Solid Edge part; units mm, degrees
sketch "Sketch1" plane through (0, 0, 0) normal (0, 0, 1) x (1, 0, 0)
  line L0 (70, -35) -> (70, 35)
  line L1 (70, 35) -> (34, 35)
  line L2 (34, 35) -> (34, 105)
  line L3 (34, 105) -> (-34, 105)
  line L4 (-34, 105) -> (-34, 35)
  line L5 (-34, 35) -> (-70, 35)
  line L6 (-70, 35) -> (-70, -35)
  line L7 (-40, -35) -> (-70, -35)
  line L8 (-40, -80) -> (-40, -35)
  line L9 (40, -80) -> (-40, -80)
  line L10 (40, -35) -> (40, -80)
  line L11 (70, -35) -> (40, -35)
  dimension "D1" = 70
  dimension "D2" = 70
  dimension "D3" = 40
  dimension "D4" = 70
  dimension "D5" = 34
extrude "Ajout_matière_2" add sketch "Sketch1" along normal blind 3
sketch "Sketch2" plane through (0, -7.5, 3) normal (0, 0, 1) x (0, -1, 0)
  line L0 (-12.5, 55) -> (-2.5, 55)
  line L1 (-2.5, 55) -> (-2.5, 52)
  line L2 (-2.5, 52) -> (-12.5, 52)
  line L3 (-12.5, 52) -> (-12.5, 55)
  line L4 (-13.5, 25) -> (-1.5, 25)
  line L5 (-1.5, 25) -> (-1.5, 38)
  line L6 (-1.5, 38) -> (-13.5, 38)
  line L7 (-13.5, 38) -> (-13.5, 25)
  circle A0 centre (37.5, 27.5) radius 2
  line L8 (-12.5, 59) -> (-2.5, 59)
  line L9 (-2.5, 59) -> (-2.5, 62)
  line L10 (-2.5, 62) -> (-12.5, 62)
  line L11 (-12.5, 62) -> (-12.5, 59)
  dimension "D1" = 2.5
  dimension "D2" = 2.5
  dimension "D3" = 37.5
  dimension "D4" = 37.5
  dimension "D5" = 1.5
  dimension "D6" = 1.5
  dimension "D7" = 1.5
extrude "Cutout1" cut sketch "Sketch2" against normal blind 6.2892
sketch "Sketch3" plane through (0, -7.5, 3) normal (0, 0, 1) x (0, -1, 0)
  line L0 (-42.5, 52) -> (-42.5, 62)
  line L1 (-42.5, 62) -> (-32.5, 62)
  line L2 (-32.5, 62) -> (-32.5, 52)
  line L3 (-32.5, 52) -> (-42.5, 52)
  dimension "D1" = 42.5
extrude "Enlèvement_matière_13" cut sketch "Sketch3" against normal blind 16.2231
sketch "Sketch4" plane through (0, -7.5, 3) normal (0, 0, 1) x (0, -1, 0)
  circle A0 centre (-22.5, 60.5) radius 1.5
  circle A1 centre (-22.5, 53.5) radius 1.5
extrude "Enlèvement_matière_14" cut sketch "Sketch4" against normal blind 7.9074
mirror "Mirror1" about plane through (0, 0, 0) normal (0, -1, 0) of "Enlèvement_matière_13", "Enlèvement_matière_14"
mirror "Mirror2" about plane through (0, 0, 0) normal (1, 0, 0) of "Enlèvement_matière_14", "Mirror1", "Enlèvement_matière_13", "Cutout1"
sketch "Sketch5" plane through (0, 10, 3) normal (0, 0, 1) x (0, 1, 0)
  circle A0 centre (66.03, 24.3) radius 1.6
  circle A1 centre (64.76, -24.29) radius 1.6
  circle A2 centre (13.96, 19.22) radius 1.6
  circle A3 centre (13.96, -9.05) radius 1.6
  dimension "D1" = 66.03
extrude "Cutout9" cut sketch "Sketch5" against normal blind 7.5802
sketch "Sketch6" plane through (0, 12.5, 3) normal (0, 0, 1) x (0, 1, 0)
  circle A0 centre (87.5, 29) radius 1.5
  circle A1 centre (87.5, -29) radius 1.5
  circle A2 centre (85.5, -11) radius 3.5
  dimension "D1" = 87.5
  dimension "D2" = 87.5
extrude "Enlèvement_matière_23" cut sketch "Sketch6" against normal blind 9.1147
properties part number "25" material "MDF 3mm"
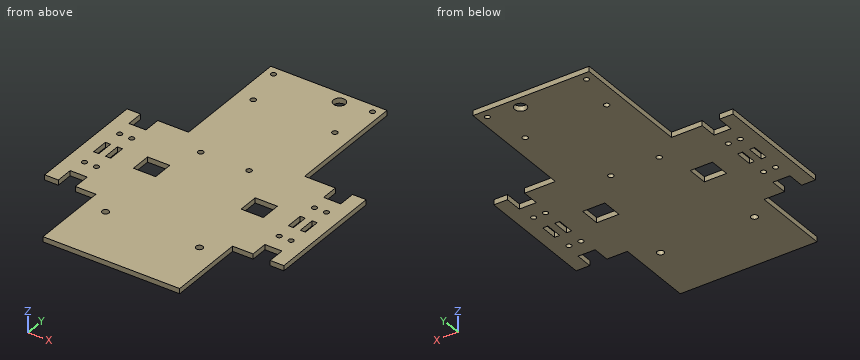
Design review of the part built by this model. Coordinates are the model's own, in mm. Round coordinates to 2 decimals unless told otherwise and drop trailing zeros. Loops run counter-clockwise (first coordinate to the right, second up) from the corner with the lowest first, then second, coordinate; pieces in that order, holes last. Notation, with made-up numbers: M 77.5,-5.75 L 124.5,-5.75 A14 ccw 124.5,-0.75 Z; hole C 25.25,8 d2. An arc over 180 degrees is marked long. Answer as a JSON object with one key per item and string values.
Item 1: We need section D-D on x = -43. Give the boundary of the cut face in (y, z).
Answer sheet:
{"outline": "M -35,0 L 35,0 L 35,3 L -35,3 Z"}
Item 2: Clearance check with flat-ended pins moving along their axes: P1, Ø0.9, axis at x = -48, z = 1.5, coming from the -Y side; P2, Ø0.9, axis at x = 53, z = 2, coming from the +Y side; P3, Ø0.9, axis at x = -53.5, z = 1, coming from the -Y side; P4, Ø6, axis at x = 25, y = -15.5, coming from the -Z side. State where each tip first meets the part, or that it passes through.
Answer sheet:
{"P1": "stops at y = -35", "P2": "stops at y = 25", "P3": "stops at y = -25", "P4": "stops at z = 0"}
Item 3: We need section A-A on y = 1. Give the boundary of the cut face in (x, z).
Answer sheet:
{"outline": "M -70,0 L -62,0 L -62,3 L -70,3 Z; M -59,0 L -55,0 L -55,3 L -59,3 Z; M -52,0 L -38,0 L -38,3 L -52,3 Z; M -25,0 L 25,0 L 25,3 L -25,3 Z; M 38,0 L 52,0 L 52,3 L 38,3 Z; M 55,0 L 59,0 L 59,3 L 55,3 Z; M 62,0 L 70,0 L 70,3 L 62,3 Z"}
Item 4: Wall thickness on L1, parallel to X at y = 15, z = 2.45; L2, parallel to Y at x = -60.5, z = 1.35; L3, parallel to Y at x = 9.05, z = 0.7: over which ranges is each line inside the solid? List them lowest first. Write a range as from..to.
Answer sheet:
{"L1": "x = -70..-62, -59..-55, -52..52, 55..59, 62..70", "L2": "y = -25..-16.5, -13.5..-5, 5..13.5, 16.5..25", "L3": "y = -80..22.36, 25.56..95.09, 100.91..105"}
Item 5: We need section B-B on y = -45. Give the boundary of the cut face in (x, z).
Answer sheet:
{"outline": "M -40,0 L -29.5,0 L -29.5,3 L -40,3 Z; M -25.5,0 L 25.5,0 L 25.5,3 L -25.5,3 Z; M 29.5,0 L 40,0 L 40,3 L 29.5,3 Z"}
Item 6: We need section C-C on z = 0.5. State how many separate pieces and enclosed holes the cut face has, and give its area (3 significant figures).
Answer sheet:
{"separate pieces": "1", "enclosed holes": "23", "area": "17,200 mm^2"}
